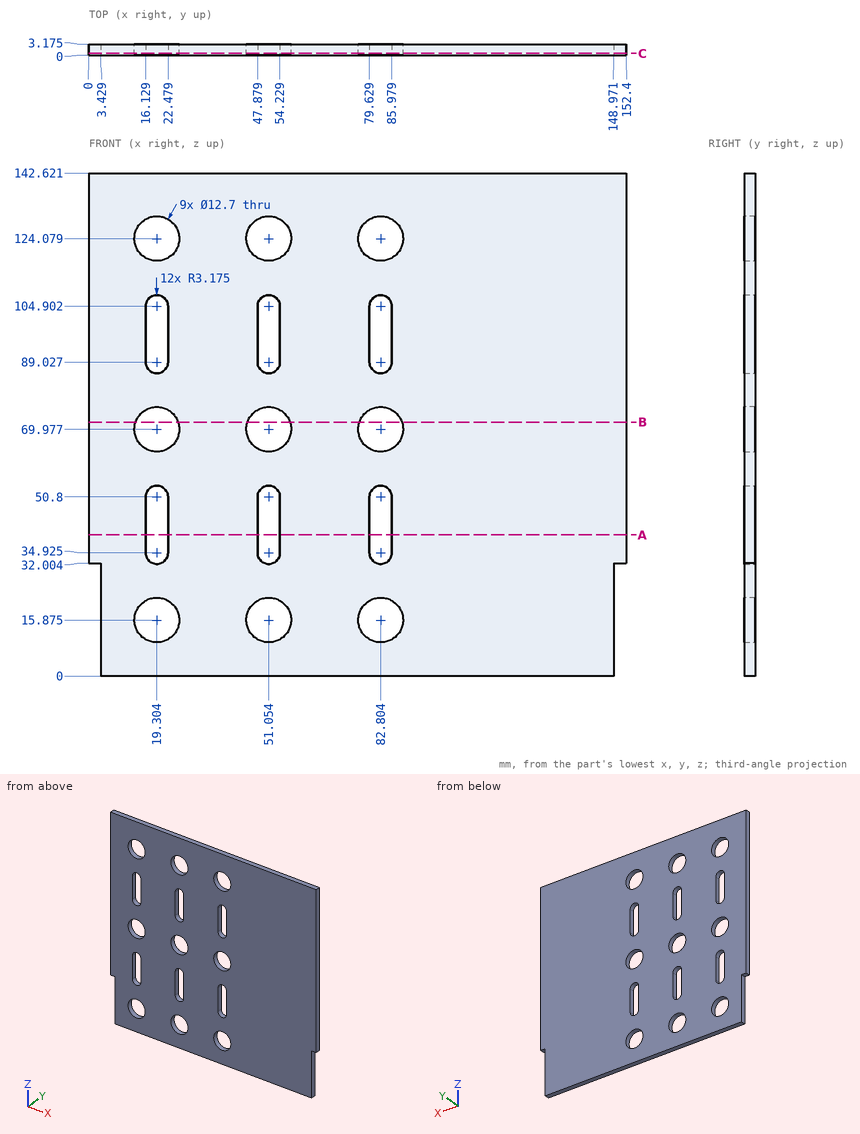
Can you work these out from the drawing? Everything is in mm from the part's minimum corner. Give positions to 0.01 mm unless a question says otherwise; leave off trailing zeros. Order: outer loops, then holes, each group sorted by start corner. A loop starts at its lowest first (then second) coordinate and runs counter-clockwise, first axis right, second up. Notation, with made-up numbers: M 24,72.5 L 70,72.5 A12 ccw 70,95.5 Z; hole C 83.25,68.5 d8. An arc over 180 degrees is marked long. Use a Markdown table: item, result. Add a question column.
Item 1: Suppose I cut it at C-C (y = 0.55). Count the separate pieces of the cut face and the enclosed holes in it, then the cut area to 3 significant figures.
Item 2: If I drill on L1, parallel to Z at x = 82.5, y = 1.05; L2, parallel to X at y = 2.7, z = 89.5; L3, parallel to X at y = 1.4, z = 74, over which ranges is the centre line in solid material (lowest first)? Write a range as [from, to].
Item 3: Suppose I cut it at A-A (z = 40). List the corners of the cut face in (x, y) for me (3 decimals).
Item 4: Will these pins go through, and if not, where does the flat tip stop? pin 1 (4 mm diameter, centred on x = 103.5, z = 71.5, fed in from -Y); pin 2 (1 mm diameter, centred on x = 1.5, y = 1.5, fed in from -Z).
Item 5: Suppose I cut it at B-B (z = 72). List the corners of the cut face in (x, y) for me (3 decimals).
Answer sheet:
| question | item | result |
|---|---|---|
| 1 | separate pieces | 1 |
| 1 | enclosed holes | 15 |
| 1 | area | 19,600 mm² |
| 2 | L1 | z = [0, 9.53], [22.22, 31.76], [53.96, 63.63], [76.32, 85.87], [108.06, 117.74], [130.42, 142.62] |
| 2 | L2 | x = [0, 16.13], [22.48, 47.88], [54.23, 79.63], [85.98, 152.4] |
| 2 | L3 | x = [0, 14.39], [24.22, 46.14], [55.97, 77.89], [87.72, 152.4] |
| 3 | outline | M 0,0 L 16.129,0 L 16.129,3.175 L 0,3.175 Z; M 22.479,0 L 47.879,0 L 47.879,3.175 L 22.479,3.175 Z; M 54.229,0 L 79.629,0 L 79.629,3.175 L 54.229,3.175 Z; M 85.979,0 L 152.4,0 L 152.4,3.175 L 85.979,3.175 Z |
| 4 | pin 1 | stops at y = 0 |
| 4 | pin 2 | stops at z = 32 |
| 5 | outline | M 0,0 L 13.285,0 L 13.285,3.175 L 0,3.175 Z; M 25.323,0 L 45.035,0 L 45.035,3.175 L 25.323,3.175 Z; M 57.073,0 L 76.785,0 L 76.785,3.175 L 57.073,3.175 Z; M 88.823,0 L 152.4,0 L 152.4,3.175 L 88.823,3.175 Z |
